Design review of the part built by this model. Coordinates are the model's own, in mm. A direction names the side the tool comes from. Round coordinates to 2 decimals unless told otherwise and drop trailing zeros. Loops run counter-clockwise (first coordinate to the right, second up) from the corner with the lowest first, then second, coordinate; pieces in that order, holes last. Notation, with made-up numbers: (65.25, 32.25) -> (73.25, 32.25) arc R24 cw to (73.25, 65.25) -> close; hole circle Ø1 at (77.5, -39.75). An arc over 180 degrees is marked (long way). Answer as CSV lines item,"result". Start each with the question number.
(1) Machinability: for faces 1 (the face through (-39.22, 19.35, -39.97)), 2 (the face through (-76.905, 14.79, -0.867)), which of the approach directions +Z, -Z, +X, -X, +Y, -Y give a long, thin tool a straight path to every point of the face, cutting with its end or side? Answer none if there is none.
(2) To check wall thickness, follow line 1 (X direction, y = 3, z = 3); line 2 (X direction, y = 14.75, z = 73); line 3 (Z direction, x = 39, y = 15.25). State the ranges of each line that lie inside material, in increasing order. Write a range as from..to.
(3) For P1, Ø2, axis at x = -0.5, z = -5.5, coming from the +Y side; P2, Ø1, axis at y = 3.5, z = -42, coming from the +X side; P3, Ø12, axis at y = 4, z = -64.5, coming from the +X side, all flat-tipped, find the tip position at first contact; note any pin that passes through.
(4) Take a section at A-A, the plane x = 0. Write out the cut boundary in (y, z).
(5) Draft analysis for pull direction Z (two halves, no side actions). For faces 3 (the face through (-85, 15, 0)), 4 (the face through (60.052, 19.353, 9.824)), 5 (the face through (-1, 0, -1)), state which applies: +Z half, -Z half, draft (parallel to the pull), parting line (faces both ways), or undercut.
(6) Take a section at B-B, the plane y = 6.75. Write out the cut boundary in (x, z).
(7) Take a section at C-C, the plane z = 73. Write out the cut boundary in (x, y), and give its area (3 significant figures).
(8) Take a section at D-D, the plane x = -73. Write out the cut boundary in (y, z), and give its area (3 significant figures).
from build123d import *

# Parameters (mm, degrees)
SKETCH1_R           = 4
SKETCH1_R_2         = 65
BOSS_EXTRUDE1_DEPTH = 30
SHELL1_START        = 9
SHELL1_DEPTH        = 21


# Read off the part's stored shape, not the designer's step: Shell1
with BuildPart() as part:
    # Sketch1 → Boss-Extrude1 (new body)
    # profile 1 of 5: a face of its own
    with BuildSketch(Plane(origin=(0, 0, 0), x_dir=(1, 0, 0), z_dir=(0, 1, 0))):
        with BuildLine():
            ThreePointArc((-61.923076923, 19.761896275), (-85, 0), (-61.923076923, -19.761896275))
            ThreePointArc((-61.923076923, -19.761896275), (-65, 0), (-61.923076923, 19.761896275))
        make_face()
        with Locations(Location((-73, 0, 0), (0, 0, 270))):
            Circle(SKETCH1_R, mode=Mode.SUBTRACT)
    # profile 2 of 5: a face of its own
    with BuildSketch(Plane(origin=(0, 0, 0), x_dir=(1, 0, 0), z_dir=(0, 1, 0))):
        with BuildLine():
            ThreePointArc((-19.761896275, -61.923076923), (0, -85), (19.761896275, -61.923076923))
            ThreePointArc((19.761896275, -61.923076923), (0, -65), (-19.761896275, -61.923076923))
        make_face()
        with Locations(Location((0, -73, 0), (0, 0, 270))):
            Circle(SKETCH1_R, mode=Mode.SUBTRACT)
    # profile 3 of 5: a face of its own
    with BuildSketch(Plane(origin=(0, 0, 0), x_dir=(1, 0, 0), z_dir=(0, 1, 0))):
        Circle(SKETCH1_R_2)
    # profile 4 of 5: a face of its own
    with BuildSketch(Plane(origin=(0, 0, 0), x_dir=(1, 0, 0), z_dir=(0, 1, 0))):
        with BuildLine():
            ThreePointArc((65, 0), (64.226162893, -10), (61.923076923, -19.761896275))
            ThreePointArc((61.923076923, -19.761896275), (85, 0), (61.923076923, 19.761896275))
            ThreePointArc((61.923076923, 19.761896275), (64.226162893, 10), (65, 0))
        make_face()
        with Locations(Location((73, 0, 0), (0, 0, 270))):
            Circle(SKETCH1_R, mode=Mode.SUBTRACT)
    # profile 5 of 5: a face of its own
    with BuildSketch(Plane(origin=(0, 0, 0), x_dir=(1, 0, 0), z_dir=(0, 1, 0))):
        with BuildLine():
            ThreePointArc((-19.761896275, 61.923076923), (0, 65), (19.761896275, 61.923076923))
            ThreePointArc((19.761896275, 61.923076923), (0, 85), (-19.761896275, 61.923076923))
        make_face()
        with Locations(Location((0, 73, 0), (0, 0, 270))):
            Circle(SKETCH1_R, mode=Mode.SUBTRACT)
    extrude(amount=BOSS_EXTRUDE1_DEPTH)

    # Shell1 outline → Shell1 (cut)
    with BuildSketch(Plane(origin=(0, 0, 0), x_dir=(1, 0, 0), z_dir=(0, 1, 0)).offset(SHELL1_START)):
        with BuildLine():
            ThreePointArc((-66, -10.95445115), (-60.127949817, -9.862207005), (-55.692307692, -5.86232581))
            ThreePointArc((-55.692307692, -5.86232581), (-39.597979746, -39.597979746), (-5.86232581, -55.692307692))
            ThreePointArc((-5.86232581, -55.692307692), (-9.862207005, -60.127949817), (-10.95445115, -66))
            ThreePointArc((-10.95445115, -66), (0, -60), (10.95445115, -66))
            ThreePointArc((10.95445115, -66), (9.862207005, -60.127949817), (5.86232581, -55.692307692))
            ThreePointArc((5.86232581, -55.692307692), (39.597979746, -39.597979746), (55.692307692, -5.86232581))
            ThreePointArc((55.692307692, -5.86232581), (60.127949817, -9.862207005), (66, -10.95445115))
            ThreePointArc((66, -10.95445115), (60, 0), (66, 10.95445115))
            ThreePointArc((66, 10.95445115), (60.127949817, 9.862207005), (55.692307692, 5.86232581))
            ThreePointArc((55.692307692, 5.86232581), (39.597979746, 39.597979746), (5.86232581, 55.692307692))
            ThreePointArc((5.86232581, 55.692307692), (9.862207005, 60.127949817), (10.95445115, 66))
            ThreePointArc((10.95445115, 66), (0, 60), (-10.95445115, 66))
            ThreePointArc((-10.95445115, 66), (-9.862207005, 60.127949817), (-5.86232581, 55.692307692))
            ThreePointArc((-5.86232581, 55.692307692), (-39.597979746, 39.597979746), (-55.692307692, 5.86232581))
            ThreePointArc((-55.692307692, 5.86232581), (-60.127949817, 9.862207005), (-66, 10.95445115))
            ThreePointArc((-66, 10.95445115), (-60, 0), (-66, -10.95445115))
        make_face()
    extrude(amount=SHELL1_DEPTH, mode=Mode.SUBTRACT)


solid = part.part
The answers:
1,face 1,"+Y"
1,face 2,"+Y, -Y"
2,line 1,"-84.77..-75.65, -70.35..70.35, 75.65..84.77"
2,line 2,"-18.33..-4, 4..18.33"
2,line 3,"-52..-40.19, 40.19..52"
3,P1,"y = 9"
3,P2,"x = 50.03"
3,P3,"x = 28.33"
4,outline,"(0, -85) -> (30, -85) -> (30, -77) -> (0, -77) -> close; (0, -69) -> (30, -69) -> (30, -60) -> (9, -60) -> (9, 60) -> (30, 60) -> (30, 69) -> (0, 69) -> close; (0, 77) -> (30, 77) -> (30, 85) -> (0, 85) -> close"
5,face 3,"parting line"
5,face 4,"undercut"
5,face 5,"draft"
6,outline,"(-61.92, -19.76) arc R65 ccw to (-19.76, -61.92) arc R20 ccw (long way) to (19.76, -61.92) arc R65 ccw to (61.92, -19.76) arc R20 ccw (long way) to (61.92, 19.76) arc R65 ccw to (19.76, 61.92) arc R20 ccw (long way) to (-19.76, 61.92) arc R65 ccw to (-61.92, 19.76) arc R20 ccw (long way) to start; hole circle Ø8 at (-73, 0); hole circle Ø8 at (0, -73); hole circle Ø8 at (0, 73); hole circle Ø8 at (73, 0)"
7,outline,"(-18.33, 0) -> (-4, 0) -> (-4, 30) -> (-18.33, 30) -> close; (4, 0) -> (18.33, 0) -> (18.33, 30) -> (4, 30) -> close"
7,area,"860 mm²"
8,outline,"(0, -18.33) -> (30, -18.33) -> (30, -4) -> (0, -4) -> close; (0, 4) -> (30, 4) -> (30, 18.33) -> (0, 18.33) -> close"
8,area,"860 mm²"
